Autodesk Fusion 360 part; units mm, degrees
sketch "Sketch1" plane through (0, 0, 0) normal (0, 0, 1) x (1, 0, 0)
  line L0 (25, 4.5) -> (-25, 4.5)
  line L1 (-25, 4.5) -> (-25, -4.5)
  line L2 (-25, -4.5) -> (25, -4.5)
  line L3 (25, -4.5) -> (25, 4.5)
  line L4 (25, 4.5) -> (-25, -4.5) construction
  line L5 (-25, 4.5) -> (25, -4.5) construction
  dimension "d1" = 50
  dimension "d2" = 9
extrude "Extrude1" add sketch "Sketch1" along normal blind 2
fillet "Fillet1" radius 2.5 4 edges at (-25, -4.5, 1) (-25, 4.5, 1) (25, -4.5, 1) (25, 4.5, 1)
sketch "Sketch2" plane through (0, 0, 2) normal (0, 0, 1) x (-1, 0, 0)
  arc A0 (-25, -2) -> (-22.5, -4.5) centre (-22.5, -2) ccw
  line L0 (-22.5, -4.5) -> (22.5, -4.5)
  arc A1 (22.5, -4.5) -> (25, -2) centre (22.5, -2) ccw
  line L1 (22.5, 4.5) -> (-22.5, 4.5)
  line L2 (25, -2) -> (25, 2)
  arc A2 (25, 2) -> (22.5, 4.5) centre (22.5, 2) ccw
  arc A3 (-22.5, 4.5) -> (-25, 2) centre (-22.5, 2) ccw
  line L3 (-25, 2) -> (-25, -2)
  line L4 (25, 0) -> (-25, 0) construction
  line L5 (25, 0) -> (20.5, 0)
  line L6 (-25, 0) -> (-20.5, 0)
  circle A4 centre (20.5, 0) radius 2.7
  circle A5 centre (-20.5, 0) radius 2.7
  dimension "d11" = 4.5
  dimension "d12" = 4.5
  dimension "d13" = 5.4
  dimension "d14" = 5.4
extrude "Extrude2" cut sketch "Sketch2" against normal blind 2 contours A4 | A5
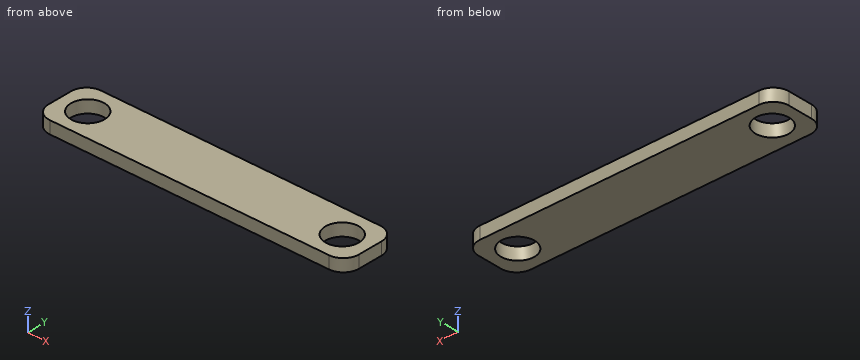
Read the model definition and answer for the solid it produces. Units are mm, in the model's axes. Give positions to 0.01 mm unless a question says otherwise; leave off trailing zeros. Loops run counter-clockwise (first coordinate to the right, second up) from the corner with the lowest first, then second, coordinate; pieces in that order, holes last.
Item 1: The part is cut by section C-C (y = 0). Write down the section's boundary in (x, z), and give its area (3 significant figures).
Item 2: The part is cut by section A-A (x = -20.5). Write down the section's boundary in (y, z), and give its area (3 significant figures).
Item 3: Find the intervals of material crossed by line 1 along X through (y, z) = (0, 0.95); line 2 along Y through (x, z) = (-20.5, 0.65); line 3 along X through (y, z) = (2, 0.65), in increasing order.
Item 4: The part is cut by section D-D (x = 20). Write down the section's boundary in (y, z).
Item 5: The part is cut by section B-B (z = 1). Write down the section's boundary in (x, y).
Item 6: This flat-tipped pin is pushed along its axis until it touches: pin 1 Ø1 at (y, z) = (-3, 1) entering from +X. Where does it stop, or does it pass through?
Taken from the geometry:
1. outline: (-25, 0) - (-23.2, 0) - (-23.2, 2) - (-25, 2) - close; (-17.8, 0) - (17.8, 0) - (17.8, 2) - (-17.8, 2) - close; (23.2, 0) - (25, 0) - (25, 2) - (23.2, 2) - close
1. area: 78.4 mm2
2. outline: (-4.5, 0) - (-2.7, 0) - (-2.7, 2) - (-4.5, 2) - close; (2.7, 0) - (4.5, 0) - (4.5, 2) - (2.7, 2) - close
2. area: 7.20 mm2
3. line 1: x = -25 to -23.2, -17.8 to 17.8, 23.2 to 25
3. line 2: y = -4.5 to -2.7, 2.7 to 4.5
3. line 3: x = -25 to -22.31, -18.69 to 18.69, 22.31 to 25
4. outline: (-4.5, 0) - (-2.65, 0) - (-2.65, 2) - (-4.5, 2) - close; (2.65, 0) - (4.5, 0) - (4.5, 2) - (2.65, 2) - close
5. outline: (-25, -2) arc R2.5 ccw to (-22.5, -4.5) - (22.5, -4.5) arc R2.5 ccw to (25, -2) - (25, 2) arc R2.5 ccw to (22.5, 4.5) - (-22.5, 4.5) arc R2.5 ccw to (-25, 2) - close; hole circle Ø5.4 at (-20.5, 0); hole circle Ø5.4 at (20.5, 0)
6. pin 1: stops at x = 24.95
